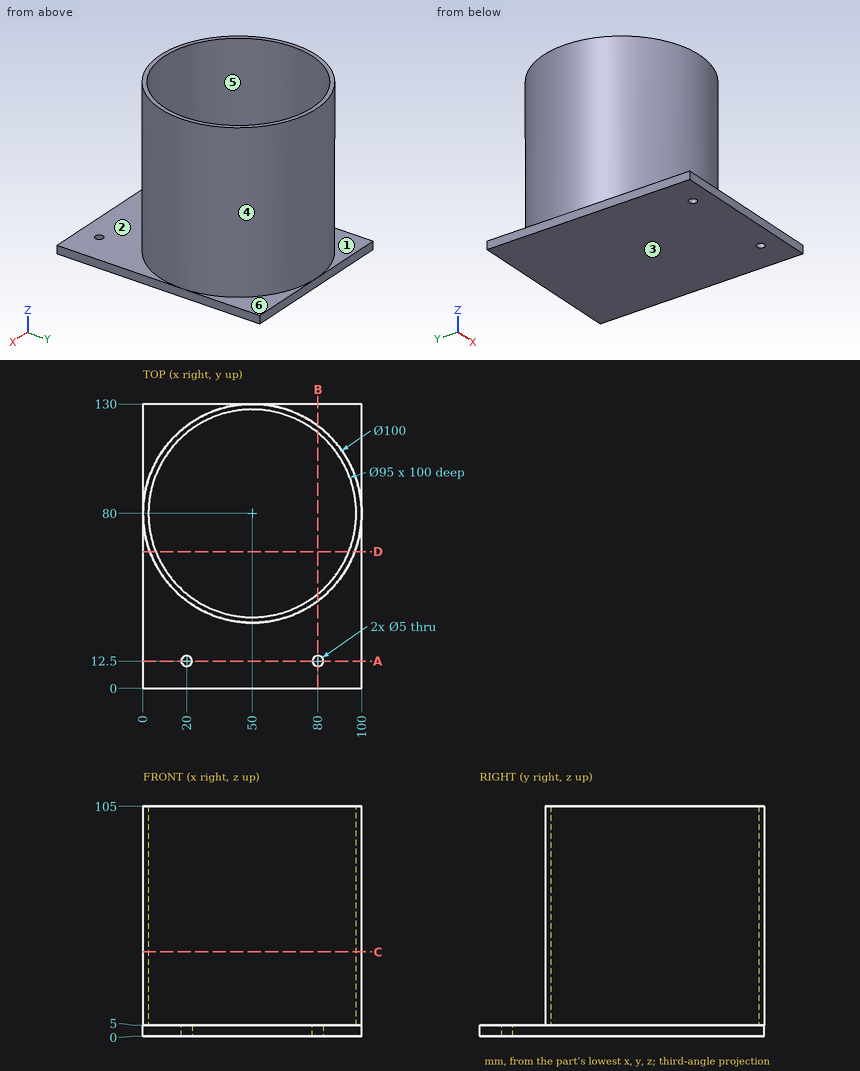
Drawing for the job (mm, zero at the part's lowest x, y, z). A direction names the side the tool comes from. Round coordinates to 2 decimals unless told otherwise and drop trailing zeros. Loops run counter-clockwise (first coordinate to the right, second up) from the corner with the lowest first, then second, coordinate; pieces in that order, holes last. Notation, with made-up numbers: (83.5, -27) -> (127.5, -27) arc R14 ccw to (127.5, 0) -> close; hole circle Ø6 at (23.25, 9). An arc over 180 degrees is marked (long way). Answer in a Markdown table with one row per item.
Item 1: Drill centre lines: L1, parallel to Y at x = 20, z = 1.95; L2, parallel to Z at x = 36.5, y = 48; L3, parallel to X at y = 61.5, z = 77. Where is each one in solid material? Low to high. Write a range as [from, to].
Answers below:
| item | result |
|---|---|
| L1 | y = [0, 10], [15, 130] |
| L2 | z = [0, 5] |
| L3 | x = [3.55, 6.25], [93.75, 96.45] |
Item 2: Saw through at A-A (y = 12.5). Write the cut outline in (x, z), and give its area (3 significant figures).
Answers below:
| item | result |
|---|---|
| outline | (0, 0) -> (17.5, 0) -> (17.5, 5) -> (0, 5) -> close; (22.5, 0) -> (77.5, 0) -> (77.5, 5) -> (22.5, 5) -> close; (82.5, 0) -> (100, 0) -> (100, 5) -> (82.5, 5) -> close |
| area | 450 mm² |
Item 3: Which spindle directions (+Z, -Z, +X, -X, +Y, -Y) get a long thin tool onto all of the face, cutting with end or side? Do the marked faces 1, 2 and 3. Say none if no direction does.
Answers below:
| item | result |
|---|---|
| face 1 | +Z, -X, +Y |
| face 2 | +Z, -Y |
| face 3 | -Z, +X, -X, +Y, -Y |
Item 4: Saw through at C-C (z = 38.5). Write the cut outline in (x, y), and give its area (3 significant figures).
Answers below:
| item | result |
|---|---|
| outline | circle Ø100 at (50, 80); hole circle Ø95 at (50, 80) |
| area | 766 mm² |
Item 5: Mould opens along Y. For the marked faces 4, 5 and 6 say: +Y half, -Y half, draft (parallel to the pull), parting line (faces both ways), or undercut.
Answers below:
| item | result |
|---|---|
| face 4 | parting line |
| face 5 | undercut |
| face 6 | draft |
Item 6: Saw through at D-D (y = 62.5). Write the cut outline in (x, z), and give its area (3 significant figures).
Answers below:
| item | result |
|---|---|
| outline | (0, 0) -> (100, 0) -> (100, 5) -> (96.84, 5) -> (96.84, 105) -> (94.16, 105) -> (94.16, 5) -> (5.84, 5) -> (5.84, 105) -> (3.16, 105) -> (3.16, 5) -> (0, 5) -> close |
| area | 1,040 mm² |
Item 7: Saw through at B-B (x = 80). Write the cut outline in (y, z).
Answers below:
| item | result |
|---|---|
| outline | (0, 0) -> (10, 0) -> (10, 5) -> (0, 5) -> close; (15, 0) -> (130, 0) -> (130, 5) -> (120, 5) -> (120, 105) -> (116.83, 105) -> (116.83, 5) -> (43.17, 5) -> (43.17, 105) -> (40, 105) -> (40, 5) -> (15, 5) -> close |
Item 8: Pin check, flat tips, straight feed: pin 1 (12 mm diameter, centred on x = 67.5, y = 70.5, fed in from -Z); pin 2 (1.5 mm diameter, centred on x = 77, y = 45, fed in from +Z); pin 3 (1.5 mm diameter, centred on y = 63.5, z = 63.5, fed in from -X); pin 4 (1 mm diameter, centred on y = 36.5, z = 87.5, fed in from -X). Stop position of each tip, or through.
Answers below:
| item | result |
|---|---|
| pin 1 | stops at z = 0 |
| pin 2 | stops at z = 5 |
| pin 3 | stops at x = 2.55 |
| pin 4 | stops at x = 24.49 |
